The listing builds one solid part. Answer for the finished solid, in the listing's coordinates (mm). Face numbers are marked on the shaded views. A direction names the side the tool comes from. Give positions to 0.01 mm unless a question says otherwise; leave off trailing zeros. Write each loop counter-clockwise with the first axis right and the second up, starting at its lowest first coordinate (ties: lowest second). Pieces come first, ordered by that corner, then holes.
```python
from build123d import *

# Parameters (mm, degrees)
SKETCH1_R           = 2.5
SKETCH1_R_2         = 6.5
SKETCH1_R_3         = 1.8
BOSS_EXTRUDE1_DEPTH = 3
BOSS_EXTRUDE2_DEPTH = 39
BOSS_EXTRUDE3_DEPTH = 39
CUT_EXTRUDE1_DEPTH  = 3
BOSS_EXTRUDE4_DEPTH = 34
BOSS_EXTRUDE5_DEPTH = 3


with BuildPart() as part:
    # Sketch1 → Boss-Extrude1 (new body)
    with BuildSketch(Plane.XY):
        with BuildLine():
            Line((-48.416861363, 3.650350453), (-11.959014769, 37.776226585))
            ThreePointArc((-11.959014769, 37.776226585), (0, 42.5), (11.959014769, 37.776226585))
            Line((11.959014769, 37.776226585), (48.416861363, 3.650350453))
            ThreePointArc((48.416861363, 3.650350453), (49.946989961, -0.726147591), (47.22369092, -4.478303104))
            Line((47.22369092, -4.478303104), (17.66776819, -19.154227328))
            ThreePointArc((17.66776819, -19.154227328), (16.856525691, -19.446371641), (16, -19.5455))
            Line((16, -19.5455), (-16, -19.5455))
            ThreePointArc((-16, -19.5455), (-16.856525691, -19.446371641), (-17.66776819, -19.154227328))
            Line((-17.66776819, -19.154227328), (-47.22369092, -4.478303104))
            ThreePointArc((-47.22369092, -4.478303104), (-49.946989961, -0.726147591), (-48.416861363, 3.650350453))
        make_face()
        with Locations((-25, 0)):
            Circle(SKETCH1_R, mode=Mode.SUBTRACT)
        with Locations((0, -5.5455)):
            Circle(SKETCH1_R_2, mode=Mode.SUBTRACT)
        with Locations((-7.75, 14.877893759)):
            Circle(SKETCH1_R_3, mode=Mode.SUBTRACT)
        with Locations((-15.5, 1.4545)):
            Circle(SKETCH1_R_3, mode=Mode.SUBTRACT)
        with Locations((-7.75, -11.968893759)):
            Circle(SKETCH1_R_3, mode=Mode.SUBTRACT)
        with Locations(Location((7.75, -11.968893759, 0), (0, 0, 180))):
            Circle(SKETCH1_R_3, mode=Mode.SUBTRACT)
        with Locations(Location((7.75, 14.877893759, 0), (0, 0, 180))):
            Circle(SKETCH1_R_3, mode=Mode.SUBTRACT)
        with Locations(Location((15.5, 1.4545, 0), (0, 0, 180))):
            Circle(SKETCH1_R_3, mode=Mode.SUBTRACT)
        with Locations(Location((25, 0, 0), (0, 0, 180))):
            Circle(SKETCH1_R, mode=Mode.SUBTRACT)
        with Locations((-45, 0)):
            Circle(SKETCH1_R, mode=Mode.SUBTRACT)
        with Locations(Location((45, 0, 0), (0, 0, 180))):
            Circle(SKETCH1_R, mode=Mode.SUBTRACT)
        with Locations((-16, -15.7955)):
            Circle(SKETCH1_R, mode=Mode.SUBTRACT)
        with Locations(Location((16, -15.7955, 0), (0, 0, 180))):
            Circle(SKETCH1_R, mode=Mode.SUBTRACT)
    extrude(amount=BOSS_EXTRUDE1_DEPTH)

    # Sketch2 → Boss-Extrude2 (add)
    with BuildSketch(Plane.XY.offset(3)):
        with BuildLine():
            Line((-20.75, 1.4545), (-18.75, 1.4545))
            ThreePointArc((-18.75, 1.4545), (-16.237976321, 10.8295), (-9.375, 17.692476321))
            Line((-9.375, 17.692476321), (-10.375, 19.424527129))
            ThreePointArc((-10.375, 19.424527129), (-17.970027129, 11.8295), (-20.75, 1.4545))
        make_face()
        with BuildLine():
            Line((-10.375, -16.515527129), (-9.375, -14.783476321))
            ThreePointArc((-9.375, -14.783476321), (0, -17.2955), (9.375, -14.783476321))
            Line((9.375, -14.783476321), (10.375, -16.515527129))
            ThreePointArc((10.375, -16.515527129), (0, -19.2955), (-10.375, -16.515527129))
        make_face()
        with BuildLine():
            ThreePointArc((18.75, 1.4545), (16.237976321, 10.8295), (9.375, 17.692476321))
            Line((9.375, 17.692476321), (10.375, 19.424527129))
            ThreePointArc((10.375, 19.424527129), (17.970027129, 11.8295), (20.75, 1.4545))
            Line((20.75, 1.4545), (18.75, 1.4545))
        make_face()
    extrude(amount=BOSS_EXTRUDE2_DEPTH)

    # Sketch3 → Boss-Extrude3 (add)
    with BuildSketch(Plane.XY.offset(3)):
        with BuildLine():
            Line((-17.5, 29), (-17.5, 23))
            Line((-17.5, 23), (-4, 23))
            Line((-4, 23), (-4, 20))
            Line((-4, 20), (-5.378251748, 20))
            Line((-5.378251748, 20), (-9.375, 17.692476321))
            Line((-9.375, 17.692476321), (-12.918615444, 17.692476321))
            ThreePointArc((-12.918615444, 17.692476321), (-12.502444344, 19.132335325), (-13.724553319, 20))
            Line((-13.724553319, 20), (-20.5, 20))
            Line((-20.5, 20), (-20.5, 29))
            Line((-20.5, 29), (-17.5, 29))
        make_face()
    boss_extrude3 = extrude(amount=BOSS_EXTRUDE3_DEPTH)

    # Mirror1: Boss-Extrude3 across plane
    add(boss_extrude3.mirror(Plane(origin=(0, 0, 0), x_dir=(0, 0, 1), z_dir=(1, 0, 0))))

    # Sketch4 → Cut-Extrude1 (cut)
    with BuildSketch(Plane(origin=(0, 23, 0), x_dir=(1, 0, 0), z_dir=(0, 1, 0))):
        with BuildLine():
            Line((-14.224553319, -17.5), (-14.224553319, -27.5))
            ThreePointArc((-14.224553319, -27.5), (-15.724553319, -29), (-17.224553319, -27.5))
            Line((-17.224553319, -27.5), (-17.224553319, -17.5))
            ThreePointArc((-17.224553319, -17.5), (-15.724553319, -16), (-14.224553319, -17.5))
        make_face()
        with BuildLine():
            Line((14.224553319, -17.5), (14.224553319, -27.5))
            ThreePointArc((14.224553319, -27.5), (15.724553319, -29), (17.224553319, -27.5))
            Line((17.224553319, -27.5), (17.224553319, -17.5))
            ThreePointArc((17.224553319, -17.5), (15.724553319, -16), (14.224553319, -17.5))
        make_face()
    extrude(amount=-CUT_EXTRUDE1_DEPTH, mode=Mode.SUBTRACT)

    # Sketch5 → Boss-Extrude4 (add)
    with BuildSketch(Plane.XY.offset(3)):
        Polygon((-43.784396435, 23.346849864), (-43.784396435, 6.040412882), (-29.176551712, -7.739510205), (-18.086117895, -7.739510205), (-18.086117895, -4.739510205), (-27.984845454, -4.739510205), (-40.784396435, 7.334606915), (-40.784396435, 23.346849864), align=None)
    boss_extrude4 = extrude(amount=BOSS_EXTRUDE4_DEPTH)

    # Mirror2: Boss-Extrude4 across plane
    add(boss_extrude4.mirror(Plane(origin=(0, 0, 0), x_dir=(0, 0, 1), z_dir=(1, 0, 0))))

    # Sketch6 → Boss-Extrude5 (add)
    with BuildSketch(Plane(origin=(0, 0, 3), x_dir=(-1, 0, 0), z_dir=(0, 0, -1))):
        Polygon((40.784396435, 23.346849864), (40.784396435, 10.794616422), (43.784396435, 7.986506839), (43.784396435, 23.346849864), align=None)
        Polygon((-43.784396435, 23.346849864), (-43.784396435, 7.986506839), (-40.784396435, 10.794616422), (-40.784396435, 23.346849864), align=None)
    extrude(amount=BOSS_EXTRUDE5_DEPTH)


solid = part.part
```
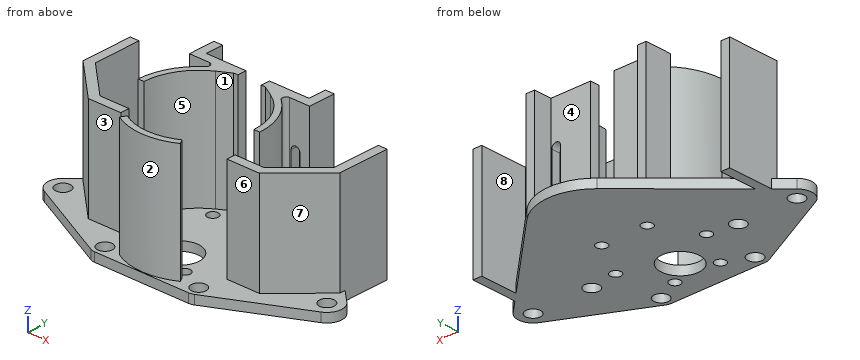
Item 1: A cutting plane is placed at C-C, the plane x = -7.75. Give the vertices of the cut face in (y, z), plus the area to 3 significant figures.
Conclusion:
outline: (-19.55, 0) - (-13.77, 0) - (-13.77, 3) - (-15.62, 3) - (-15.62, 42) - (-17.79, 42) - (-17.79, 3) - (-19.55, 3) - close; (-10.17, 0) - (13.08, 0) - (13.08, 3) - (-10.17, 3) - close; (16.68, 0) - (40.69, 0) - (40.69, 3) - (23, 3) - (23, 42) - (18.63, 42) - (18.63, 3) - (16.68, 3) - close
area: 414 mm2
Item 2: Consider probe 1 along X at (y, z) = (9.5, 28); probe 2 along X at (y, z) = (26, 11); probe 3 along X at (y, z) = (4, 12.5). Determine where each line is inside the solid, lowest interval first.
Conclusion:
probe 1: x = -43.78 to -40.78, -19.13 to -16.94, 16.94 to 19.13, 40.78 to 43.78
probe 2: x = -20.5 to -17.5, 17.5 to 20.5
probe 3: x = -41.62 to -37.25, -20.59 to -18.58, 18.58 to 20.59, 37.25 to 41.62
Item 3: Which of the six approach directions +Z, -Z, +X, -X, +Y, -Y give full straight-line access (tool end or side, diameter ignored) to the marked faces 5, 6, 7 and 8?
Conclusion:
face 5: +Z
face 6: +Z, +X, -X, -Y
face 7: +Z, +X, -Y
face 8: +Z, +Y
Item 4: A cutting plane is placed at B-B, the plane z = 24. Count the separate pieces of the cut face and the enclosed holes in it, plus the area to 3 significant figures.
Conclusion:
separate pieces: 7
enclosed holes: 0
area: 535 mm2
Item 5: A cutting plane is placed at A-A, the plane x = -25. Give the vertices of the cut face in (y, z), plus the area to 3 significant figures.
Conclusion:
outline: (-15.51, 0) - (-2.5, 0) - (-2.5, 3) - (-4.74, 3) - (-4.74, 37) - (-7.74, 37) - (-7.74, 3) - (-15.51, 3) - close; (2.5, 0) - (25.57, 0) - (25.57, 3) - (2.5, 3) - close
area: 210 mm2
Item 6: Each of these flat-tipped pins is pushed along its axis until it touches: P1, Ø3, axis at y = 26, z = 28, coming from the +X side; P2, Ø3, axis at x = -16, y = -15.8, coming from the -Z side; P3, Ø4, axis at x = 15.5, y = 1.45, coming from the +Z side; P4, Ø1.5, axis at y = 22.5, z = 30.5, coming from the -X side. Where does it stop, or does it pass through?
Conclusion:
P1: stops at x = 20.5
P2: passes through
P3: stops at z = 3
P4: stops at x = -43.78
Item 7: Determine the mould class of the marked faces 1, 2, 3 and 4 for opening direction X: pulls with the +X half, pulls with the -X half, needs draft (parallel to the pull), parting line crosses it, or undercut.
Conclusion:
face 1: undercut
face 2: parting line crosses it
face 3: needs draft
face 4: undercut
